Verification items for the finished model (mm, model axes). Face numbers are marked on the shaded views. Give positions to 0.01 mm unless a question says otherwise; leave off trailing zeros. Write each loop counter-clockwise with the first axis right and the second up, starting at its lowest first coordinate (ties: lowest second). Pieces come first, ordered by that corner, then holes.
Autodesk Inventor part; units mm, degrees
ref_plane "YZ Plane" through (0, 0, 0) normal (1, 0, 0) x (0, 1, 0)
ref_plane "XZ Plane" through (0, 0, 0) normal (0, 1, 0) x (-1, 0, 0)
ref_plane "XY Plane" through (0, 0, 0) normal (0, 0, 1) x (1, 0, 0)
sketch "Sketch1" plane through (0, 0, 0) normal (0, 1, 0) x (-1, 0, 0)
  line L0 (62.65, 0) -> (-62.65, 0)
  line L1 (0, -97.65) -> (0, 97.65)
  line L2 (44.75, -69.75) -> (-44.75, -69.75)
  line L3 (-44.75, -69.75) -> (-44.75, 69.75)
  line L4 (-44.75, 69.75) -> (44.75, 69.75)
  line L5 (44.75, 69.75) -> (44.75, -69.75)
  point P0 (0, 0)
  dimension "d0" = 89.5
  dimension "d1" = 139.5
  dimension "d2" = 69.75
  dimension "d3" = 44.75
extrude "Extrusion1" add sketch "Sketch1" along normal blind 5
sketch "Sketch2" plane through (0, 5, 0) normal (0, 1, 0) x (1, 0, 0)
  circle A0 centre (-42.375, 67.375) radius 1.625
  circle A1 centre (42.375, 67.375) radius 1.625
  circle A2 centre (42.375, -67.375) radius 1.625
  circle A3 centre (-42.375, -67.375) radius 1.625
  line L0 (44.75, -69.75) -> (44.75, 69.75)
  line L1 (44.75, 69.75) -> (-44.75, 69.75)
  line L2 (-44.75, 69.75) -> (-44.75, -69.75)
  line L3 (-44.75, -69.75) -> (44.75, -69.75)
  dimension "d6" = 3.25
  dimension "d9" = 3.25
  dimension "d12" = 3.25
  dimension "d15" = 3.25
  dimension "d19" = 2.375
  dimension "d20" = 2.375
  dimension "d21" = 2.375
  dimension "d22" = 2.375
  dimension "d23" = 2.375
  dimension "d24" = 2.375
  dimension "d25" = 2.375
  dimension "d26" = 2.375
extrude "Extrusion2" cut sketch "Sketch2" against normal blind 5 contours A0 | A1 | A2 | A3
sketch "Sketch3" plane through (0, 5, 0) normal (0, 1, 0) x (1, 0, 0)
  line L0 (-34.75, -59.75) -> (34.75, -59.75)
  line L1 (34.75, -59.75) -> (34.75, 59.75)
  line L2 (34.75, 59.75) -> (-34.75, 59.75)
  line L3 (-34.75, 59.75) -> (-34.75, -59.75)
  circle A0 centre (42.375, -67.375) radius 1.625
  circle A1 centre (-42.375, 67.375) radius 1.625
  circle A2 centre (42.375, 67.375) radius 1.625
  circle A3 centre (-42.375, -67.375) radius 1.625
  line L4 (44.75, 69.75) -> (-44.75, 69.75)
  line L5 (-44.75, 69.75) -> (-44.75, -69.75)
  line L6 (-44.75, -69.75) -> (44.75, -69.75)
  line L7 (44.75, -69.75) -> (44.75, 69.75)
  line L8 (-29.75, 54.75) -> (29.75, 54.75)
  line L9 (29.75, 54.75) -> (29.75, -54.75)
  line L10 (29.75, -54.75) -> (-29.75, -54.75)
  line L11 (-29.75, -54.75) -> (-29.75, 54.75)
  point P0 (0, 0)
  dimension "d29" = 10
  dimension "d30" = 10
  dimension "d31" = 10
  dimension "d32" = 10
  dimension "d33" = 5
  dimension "d34" = 5
  dimension "d35" = 5
  dimension "d36" = 5
extrude "Extrusion3" add sketch "Sketch3" along normal blind 5 contours L3 L2 L1 L0
properties part number "mien_top"
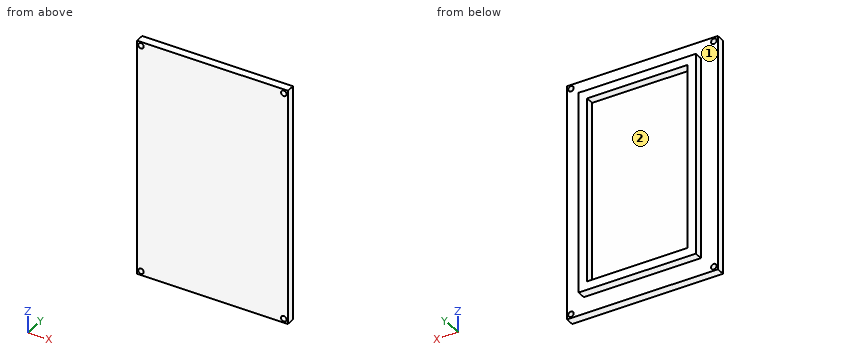
Item 1: Sectioned sample at B-B on z = 49.5. Record the cut outline in (x, y), then the cut area to 4 significant figures.
Answer key:
outline: (-44.75, 0) - (44.75, 0) - (44.75, 5) - (34.75, 5) - (34.75, 10) - (29.75, 10) - (29.75, 5) - (-29.75, 5) - (-29.75, 10) - (-34.75, 10) - (-34.75, 5) - (-44.75, 5) - close
area: 497.5 mm2
Item 2: Depth check by flat-ended pin: pin 1 (3.5 mm diameter, centred on x = -42.375, z = -67.375, fed in from +Y); pin 2 (1.5 mm diameter, centred on x = 4, y = 7, fed in from -Z); pin 3 (1.5 mm diameter, centred on y = 7.5, z = -20.5, fed in from -X). Enter the tip coordinate at first touch or a pass-through.
Answer key:
pin 1: stops at y = 5
pin 2: stops at z = -59.75
pin 3: stops at x = -34.75
Item 3: Scan lines: line 1 along Z through (x, y) = (3, 6.5); line 2 along X through (y, z) = (5.25, -40.5); line 3 along Y through (x, z) = (-21, -60). Record each from-to range of solid material in increasing order.
Answer key:
line 1: z = -59.75 to -54.75, 54.75 to 59.75
line 2: x = -34.75 to -29.75, 29.75 to 34.75
line 3: y = 0 to 5
Item 4: Release check for a two-part mould opening along X. For the marked faces 1 and 2 record: released by +X, released by -X, zero draft, split by the parting line, or undercut.
Answer key:
face 1: zero draft
face 2: undercut
Item 5: Sectioned sample at A-A on y = 7. Record the cut outline in (x, z), then the cut area to 3 significant figures.
Answer key:
outline: (-34.75, -59.75) - (34.75, -59.75) - (34.75, 59.75) - (-34.75, 59.75) - close; hole (-29.75, -54.75) - (29.75, -54.75) - (29.75, 54.75) - (-29.75, 54.75) - close
area: 1,790 mm2
Item 6: Sectioned sample at C-C on x = -32. Record the cut outline in (y, z), then the cut area to 4 significant figures.
Answer key:
outline: (0, -69.75) - (5, -69.75) - (5, -59.75) - (10, -59.75) - (10, 59.75) - (5, 59.75) - (5, 69.75) - (0, 69.75) - close
area: 1,295 mm2
Item 7: Sectioned sample at D-D on x = -2. Record the cut outline in (y, z).
Answer key:
outline: (0, -69.75) - (5, -69.75) - (5, -59.75) - (10, -59.75) - (10, -54.75) - (5, -54.75) - (5, 54.75) - (10, 54.75) - (10, 59.75) - (5, 59.75) - (5, 69.75) - (0, 69.75) - close
